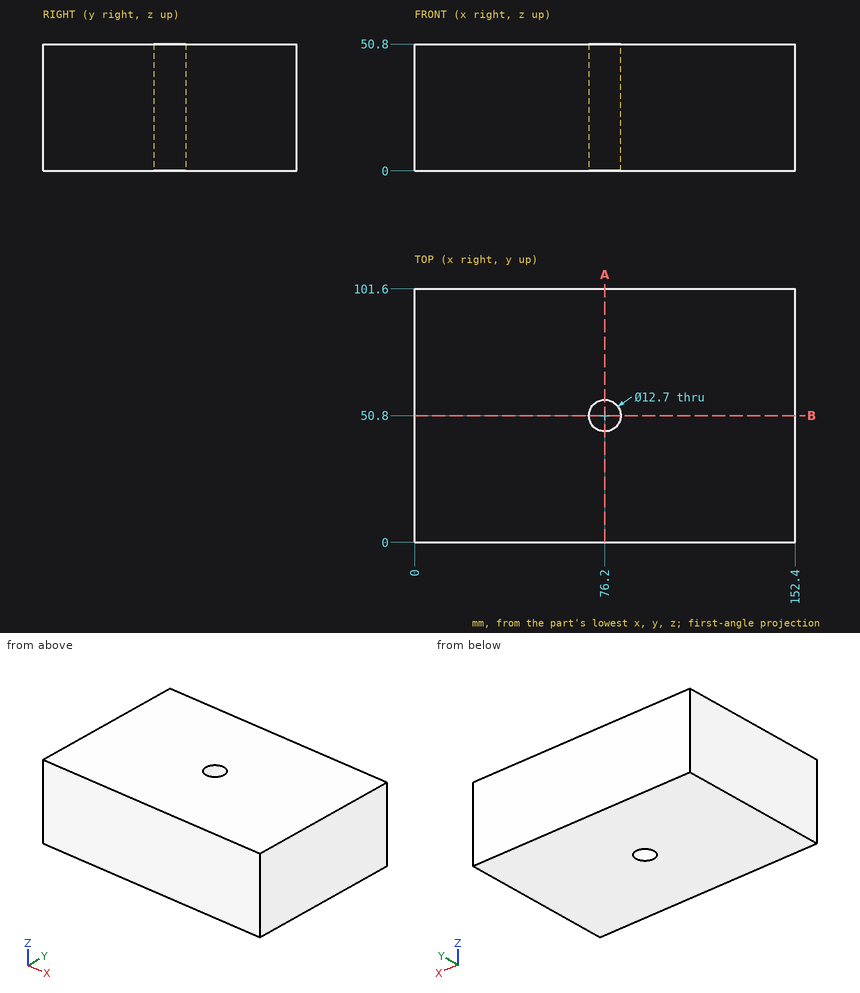
Geometry: see drawing. Coordinates: mm, zero at the bounding-box minimum. Give positions to 0.01 mm unless a question says otherwise; leave off trailing zeros. Loops run counter-clockwise (first coordinate to the right, second up) from the corner with the lowest first, then second, coordinate; pieces in that order, holes last. Notation, with made-up numbers: M -17.5,83.25 L -3.5,83.25 A21 cw -3.5,99.25 Z; hole C -12,-21.5 d5. An arc over 180 degrees is marked long. Use one line per item in the form item = value.
1. Line query: L1, parallel to Y at x = 76.2, z = 34; L2, parallel to X at y = 50.8, z = 39.5; L3, parallel to X at y = 49, z = 26. Output: solid intervals per line, ascending.
Numbers:
L1 = 0 to 44.45, 57.15 to 101.6
L2 = 0 to 69.85, 82.55 to 152.4
L3 = 0 to 70.11, 82.29 to 152.4
2. Section query B-B, the plane y = 50.8. Return the cut outline in (x, z).
Numbers:
outline = M 0,0 L 69.85,0 L 69.85,50.8 L 0,50.8 Z; M 82.55,0 L 152.4,0 L 152.4,50.8 L 82.55,50.8 Z
3. Section query A-A, the plane x = 76.2. Return the cut outline in (y, z).
Numbers:
outline = M 0,0 L 44.45,0 L 44.45,50.8 L 0,50.8 Z; M 57.15,0 L 101.6,0 L 101.6,50.8 L 57.15,50.8 Z
